```python
from build123d import *

# Parameters (mm, degrees)
SKETCH2_R           = 2.9
BOSS_EXTRUDE1_DEPTH = 2
SKETCH3_R           = 3.9
SKETCH3_R_2         = 2.9
SKETCH3_R_3         = 1.75
BOSS_EXTRUDE2_DEPTH = 2


with BuildPart() as part:
    # Sketch2 → Boss-Extrude1 (new body)
    with BuildSketch(Plane(origin=(0, 0, 0), x_dir=(1, 0, 0), z_dir=(0, 1, 0))):
        with BuildLine():
            ThreePointArc((3.9, 5.2), (0, 6.5), (-3.9, 5.2))
            Line((-3.9, 5.2), (-3.9, -5.2))
            ThreePointArc((-3.9, -5.2), (0, -6.5), (3.9, -5.2))
            Line((3.9, -5.2), (3.9, 5.2))
        make_face()
        Circle(SKETCH2_R, mode=Mode.SUBTRACT)
    extrude(amount=BOSS_EXTRUDE1_DEPTH)

    # Sketch3 → Boss-Extrude2 (add)
    with BuildSketch(Plane(origin=(0, 2, 0), x_dir=(1, 0, 0), z_dir=(0, 1, 0))):
        Circle(SKETCH3_R)
        Circle(SKETCH3_R_2, mode=Mode.SUBTRACT)
        Circle(SKETCH3_R_2)
        Circle(SKETCH3_R_3, mode=Mode.SUBTRACT)
    extrude(amount=BOSS_EXTRUDE2_DEPTH)


solid = part.part
```
The listing builds one solid part. Answer for the finished solid, in the listing's coordinates (mm). A direction names the side the tool comes from. Give positions to 0.01 mm unless a question says otherwise; leave off trailing zeros. Write each loop counter-clockwise with the first axis right and the second up, starting at its lowest first coordinate (ties: lowest second). Pieces come first, ordered by that corner, then holes. Notation, with made-up numbers: (50.25, 82) -> (81.25, 82) arc R28 ccw to (81.25, 115) -> close; hole circle Ø3 at (-5.75, -22.75). An arc over 180 degrees is marked (long way). Use one line per item in the form item = value.
1) Section B-B on y = 1.4 is taken. Write down the section's boundary in (x, z).
Result:
outline = (-3.9, -5.2) arc R6.5 ccw to (3.9, -5.2) -> (3.9, 5.2) arc R6.5 ccw to (-3.9, 5.2) -> close; hole circle Ø5.8 at (0, 0)
2) A tool of negligible diameter and unlimited length cuts with its end or side. For faces 4 (the cylindrical face through (-2.9, 1, -0.1)), 5 (the flat face through (-3, 0, -2)), 6 (the cylindrical face through (-2.87, 2.99, -2.64)), from which of +Z, -Z, +X, -X, +Y, -Y can it reach the whole face along a straight path? Write none if from no direction.
Result:
face_4 = -Y
face_5 = +Z, -Z, +X, -X, -Y
face_6 = +Y
3) Section D-D on x = -2 is taken. Write down the section's boundary in (y, z), plus the area to 3 significant figures.
Result:
outline = (0, -6.18) -> (2, -6.18) -> (2, -3.35) -> (4, -3.35) -> (4, 3.35) -> (2, 3.35) -> (2, 6.18) -> (0, 6.18) -> (0, 2.1) -> (2, 2.1) -> (2, -2.1) -> (0, -2.1) -> close
area = 29.7 mm²
4) Straight lines are drawn through the part: probe 1 along X at (y, z) = (1.5, 0); probe 2 along Z at (x, y) = (0, 1.45); probe 3 along X at (y, z) = (2.85, 0). For each, find the intervals that lie inside material, in ascending order.
Result:
probe_1 = -3.9 to -2.9, 2.9 to 3.9
probe_2 = -6.5 to -2.9, 2.9 to 6.5
probe_3 = -3.9 to -1.75, 1.75 to 3.9
5) For a pull along X with two mould halves and no side action, classify faces 1 (the flat face through (2, 4, 1)), 2 (the flat face through (-3.9, 1, 0)), 3 (the flat face through (0, 2, 2)) as +X half, -X half, draft (parallel to the pull), parting line (faces both ways), or undercut.
Result:
face_1 = draft
face_2 = -X half
face_3 = undercut
6) Section C-C on z = 1 is taken. Write down the section's boundary in (x, y), plus the area to 3 significant figures.
Result:
outline = (-3.9, 0) -> (-2.72, 0) -> (-2.72, 2) -> (-1.44, 2) -> (-1.44, 4) -> (-3.77, 4) -> (-3.77, 2) -> (-3.9, 2) -> close; (1.44, 2) -> (2.72, 2) -> (2.72, 0) -> (3.9, 0) -> (3.9, 2) -> (3.77, 2) -> (3.77, 4) -> (1.44, 4) -> close
area = 14.0 mm²
7) Section A-A on x = 0 is taken. Write down the section's boundary in (y, z), plus the area to 3 significant figures.
Result:
outline = (0, -6.5) -> (2, -6.5) -> (2, -3.9) -> (4, -3.9) -> (4, -1.75) -> (2, -1.75) -> (2, -2.9) -> (0, -2.9) -> close; (0, 2.9) -> (2, 2.9) -> (2, 1.75) -> (4, 1.75) -> (4, 3.9) -> (2, 3.9) -> (2, 6.5) -> (0, 6.5) -> close
area = 23.0 mm²
